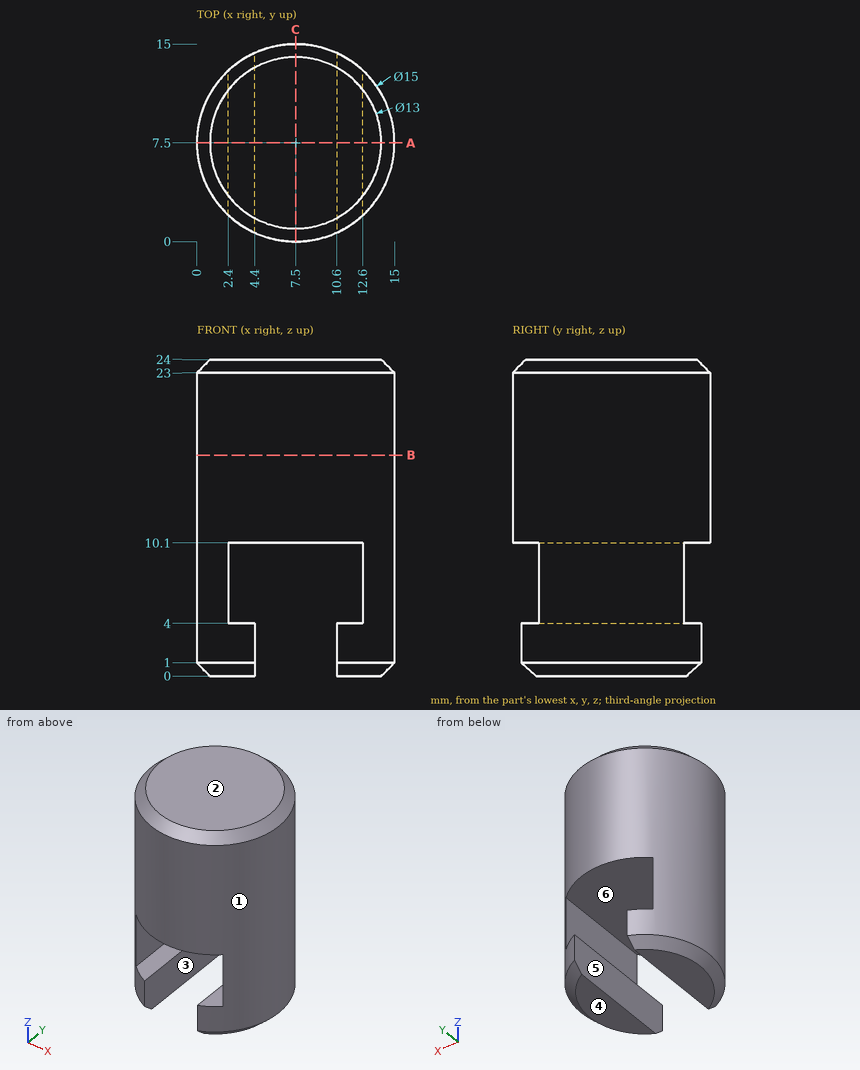
Can you work these out from the drawing? Everything is in mm from the part's minimum corner. A direction names the side the tool comes from. Give positions to 0.01 mm unless a question says otherwise; leave off trailing zeros. Order: outer loops, then holes, each group sorted by start corner. A loop starts at its lowest first (then second) coordinate and runs counter-clockwise, first axis right, second up. Notation, with made-up numbers: M 83,31.25 L 109,31.25 A25 cw 109,63.25 Z; hole C 88,52.5 d3. An arc over 180 degrees is marked long. One line per question, with ' | ' between items.
1. I want a section at A-A (y = 7.5). List the corners of the cut face in (x, z) for me.
Results:
outline: M 0,1 L 1,0 L 4.4,0 L 4.4,4 L 2.4,4 L 2.4,10.1 L 12.6,10.1 L 12.6,4 L 10.6,4 L 10.6,0 L 14,0 L 15,1 L 15,23 L 14,24 L 1,24 L 0,23 Z
2. I'm going to push flat-ended pins straight in: pin 1 (6 mm diameter, centred on y = 13.5, z = 10.5, fed in from +X); pin 2 (1 mm diameter, centred on y = 2, z = 7.5, fed in from +X); pin 3 (6 mm diameter, centred on x = 10, z = 3, fed in from -Y). Where does each tip first touch, or does it pass through?
Results:
pin 1: x = 14.37 | pin 2: x = 13.09 | pin 3: y = 0.67
3. I want a section at C-C (x = 7.5). List the corners of the cut face in (y, z) for me, and give its area (4 significant figures).
Results:
outline: M 0,10.1 L 15,10.1 L 15,23 L 14,24 L 1,24 L 0,23 Z | area: 207.5 mm²
4. I want a section at B-B (z = 16.75). List the corners of the cut face in (x, y) for me, and give its area (3 significant figures).
Results:
outline: C 7.5,7.5 d15 | area: 177 mm²
5. If I drill on line 1 (Z direction, x = 11, y = 5.75); line 2 (X direction, y = 7.75, z = 6.25); line 3 (X direction, y = 5.25, z = 8.25), over which ranges is the centre line in solid material (lowest first)?
Results:
line 1: 0 to 4, 10.1 to 24 | line 2: 0 to 2.4, 12.6 to 15 | line 3: 0.35 to 2.4, 12.6 to 14.65
6. For the marked faces 4, 5 and 6, which set-ups out of +Z, -Z, +X, -X, +Y, -Y let a thin tool reach every point of the face, with its end or its side?
Results:
face 4: -Z, +X, -X, +Y, -Y | face 5: -Z, +Y, -Y | face 6: +Y, -Y
7. We'd pull the mould along X, two halves only. Please class the marked faces 1, 2 and 3: +X half, -X half, draft (parallel to the pull), parting line (faces both ways), or undercut.
Results:
face 1: parting line | face 2: draft | face 3: undercut
